Work out the finished part from the listing and answer in its coordinate system (mm). A direction names the side the tool comes from. Coordinates: 2 decimals unless noted, no trailing zeros. Loops run counter-clockwise (first coordinate to the right, second up) from the corner with the lowest first, then second, coordinate; pieces in that order, holes last. Notation, with made-up numbers: M -25,-28 L -17,-28 A27 ccw -17,2 Z; hole C 25.25,57.25 d6. An arc over 180 degrees is marked long. Write each question's results on one line, items separated by ' | '.
```python
from build123d import *

# Parameters (mm, degrees)
CYLINDER883_R               = 1.5
CYLINDER883_DEPTH           = 20
CYLINDER884_R               = 1.5
CYLINDER884_DEPTH           = 20
CYLINDER881_R               = 1.5
CYLINDER881_DEPTH           = 20
CYLINDER885_R               = 1.5
CYLINDER885_DEPTH           = 20
BOX399_W                    = 6
BOX399_H                    = 2
BOX399_DEPTH                = 6
BOX401_W                    = 6
BOX401_H                    = 2
BOX401_DEPTH                = 6
BOX398_W                    = 6
BOX398_H                    = 2
BOX398_DEPTH                = 6
BOX402_W                    = 6
BOX402_H                    = 2
BOX402_DEPTH                = 6
CYLINDER882_R               = 4
CYLINDER882_DEPTH           = 20
CYLINDER882_PLACEMENT_ANGLE = 45
CYLINDER877_R               = 4
CYLINDER877_DEPTH           = 20
CYLINDER877_PLACEMENT_ANGLE = 45
CYLINDER880_R               = 10
CYLINDER880_DEPTH           = 40
CYLINDER878_R               = 10
CYLINDER878_DEPTH           = 40
CYLINDER879_R               = 52
CYLINDER879_DEPTH           = 8
BOX403_W                    = 108
BOX403_H                    = 36
BOX403_DEPTH                = 8
FILLET014_R                 = 12


with BuildPart() as obj1:
    # Cylinder883 → Cylinder883 (new body)
    with BuildSketch(Plane(origin=(24, -40, -5), x_dir=(1, 0, 0), z_dir=(0, -1, 0))):
        Circle(CYLINDER883_R)
    extrude(amount=CYLINDER883_DEPTH)


with BuildPart() as obj2:
    # Cylinder884 → Cylinder884 (new body)
    with BuildSketch(Plane(origin=(51, -40, 7), x_dir=(1, 0, 0), z_dir=(0, -1, 0))):
        Circle(CYLINDER884_R)
    extrude(amount=CYLINDER884_DEPTH)


with BuildPart() as obj3:
    # Cylinder881 → Cylinder881 (new body)
    with BuildSketch(Plane(origin=(-51, -40, 7), x_dir=(1, 0, 0), z_dir=(0, -1, 0))):
        Circle(CYLINDER881_R)
    extrude(amount=CYLINDER881_DEPTH)


with BuildPart() as compound773:
    # Cylinder885 → Cylinder885 (new body)
    with BuildSketch(Plane(origin=(-24, -40, -5), x_dir=(1, 0, 0), z_dir=(0, -1, 0))):
        Circle(CYLINDER885_R)
    extrude(amount=CYLINDER885_DEPTH)

    # Compound773: union obj1, obj2, obj3
    add(obj1.part)
    add(obj2.part)
    add(obj3.part)


with BuildPart() as krychle399:
    # Box399 → Box399 (new body)
    with BuildSketch(Plane(origin=(21, -47, -8), x_dir=(1, 0, 0), z_dir=(0, 0, 1))):
        with Locations((3, 1)):
            Rectangle(BOX399_W, BOX399_H)
    extrude(amount=BOX399_DEPTH)


with BuildPart() as krychle401:
    # Box401 → Box401 (new body)
    with BuildSketch(Plane(origin=(48, -45, 4), x_dir=(1, 0, 0), z_dir=(0, 0, 1))):
        with Locations((3, 1)):
            Rectangle(BOX401_W, BOX401_H)
    extrude(amount=BOX401_DEPTH)


with BuildPart() as krychle398:
    # Box398 → Box398 (new body)
    with BuildSketch(Plane(origin=(-54, -45, 4), x_dir=(1, 0, 0), z_dir=(0, 0, 1))):
        with Locations((3, 1)):
            Rectangle(BOX398_W, BOX398_H)
    extrude(amount=BOX398_DEPTH)


with BuildPart() as compound772:
    # Box402 → Box402 (new body)
    with BuildSketch(Plane(origin=(-27, -47, -8), x_dir=(1, 0, 0), z_dir=(0, 0, 1))):
        with Locations((3, 1)):
            Rectangle(BOX402_W, BOX402_H)
    extrude(amount=BOX402_DEPTH)

    # Compound772: union Krychle399, Krychle401, Krychle398
    add(krychle399.part)
    add(krychle401.part)
    add(krychle398.part)


with BuildPart() as obj4:
    # Cylinder882 → Cylinder882 (new body)
    with BuildSketch(Plane.XY):
        Circle(CYLINDER882_R)
    extrude(amount=CYLINDER882_DEPTH)


with BuildPart() as obj4_1:
    # Cylinder882 placement: moved
    add(obj4.part.moved(Location((39.6, -39.6, -10))).rotate(Axis((39.6, -39.6, -10), (0, 0, 1)), CYLINDER882_PLACEMENT_ANGLE))


with BuildPart() as compound775:
    # Cylinder877 → Cylinder877 (new body)
    with BuildSketch(Plane.XY):
        Circle(CYLINDER877_R)
    extrude(amount=CYLINDER877_DEPTH)


with BuildPart() as compound775_1:
    # Cylinder877 placement: moved
    add(compound775.part.moved(Location((-39.6, -39.6, -10))).rotate(Axis((-39.6, -39.6, -10), (0, 0, -1)), CYLINDER877_PLACEMENT_ANGLE))

    # Compound775: union obj4
    add(obj4_1.part)


with BuildPart() as obj5:
    # Cylinder880 → Cylinder880 (new body)
    with BuildSketch(Plane(origin=(-59, -17, 0), x_dir=(1, 0, 0), z_dir=(0, 0, 1))):
        Circle(CYLINDER880_R)
    extrude(amount=CYLINDER880_DEPTH)


with BuildPart() as compound774:
    # Cylinder878 → Cylinder878 (new body)
    with BuildSketch(Plane(origin=(59, -17, 0), x_dir=(1, 0, 0), z_dir=(0, 0, 1))):
        Circle(CYLINDER878_R)
    extrude(amount=CYLINDER878_DEPTH)

    # Compound774: union obj5
    add(obj5.part)


with BuildPart() as obj6:
    # Cylinder879 → Cylinder879 (new body)
    with BuildSketch(Plane.XY.offset(20)):
        Circle(CYLINDER879_R)
    extrude(amount=CYLINDER879_DEPTH)


with BuildPart() as fillet014:
    # Box403 → Box403 (new body)
    with BuildSketch(Plane(origin=(-54, -53, 20), x_dir=(1, 0, 0), z_dir=(0, 0, 1))):
        with Locations((54, 18)):
            Rectangle(BOX403_W, BOX403_H)
    extrude(amount=BOX403_DEPTH)

    # Cut400: cut obj6
    add(obj6.part, mode=Mode.SUBTRACT)


with BuildPart() as fillet014_1:
    # Cut400 placement: moved
    add(fillet014.part.moved(Location((0, 0, -20))))

    # Cut403: cut Compound774
    add(compound774.part, mode=Mode.SUBTRACT)


with BuildPart() as fillet014_2:
    # Cut403 placement: moved
    add(fillet014_1.part.moved(Location((0, 0, -8))))

    # Cut401: cut Compound775
    add(compound775_1.part, mode=Mode.SUBTRACT)

    # Cut402: cut Compound772
    add(compound772.part, mode=Mode.SUBTRACT)

    # Cut399: cut Compound773
    add(compound773.part, mode=Mode.SUBTRACT)

    # Fillet014
    fillet014_edges = [fillet014_2.edges().sort_by_distance(p)[0] for p in [
        (-54, -25.660254, -4),
        (54, -25.660254, -4),
    ]]
    fillet(fillet014_edges, radius=FILLET014_R)


solid = fillet014_2.part
```
1) Straight lines are drawn through the part: probe 1 along X at (y, z) = (-39.6, -5.25); probe 2 along X at (y, z) = (-48, -5.75); probe 3 along X at (y, z) = (-20.5, -3.5). For each, find the intervals that lie inside material, in ascending order. Write a range as [from, to].
Check result:
probe 1: [-54, -43.6], [-35.6, -33.7], [33.7, 35.6], [43.6, 54] | probe 2: [-54, -25.3], [-22.7, -20], [20, 22.7], [25.3, 54] | probe 3: [-49.63, -47.79], [47.79, 49.63]
2) For a pull along X with two mould halves and no side action, classify faces 1 (the face through (-38.071, -43.296, -4.056)), 2 (the face through (54, -42, -4)), 3 (the face through (-54, -42, -4)) as released by +X, released by -X, zero draft, split by the parting line, or undercut.
Check result:
face 1: undercut | face 2: released by +X | face 3: released by -X
3) Given pin 1 Ø1.4 at (x, z) = (25, -4.5) entering from +Y; pin 2 Ø0.6 at (x, y) = (25.5, -46) entering from -Z, each flat-ended and moving along its own axis, determine where each tip first touches the part or whether it passes through.
Check result:
pin 1: y = -47 | pin 2: z = -2
4) Find section B-B, the plane y = -27.5. Give the vertices of the cut face in (x, z).
Check result:
outline: M -53.49,-8 L -44.13,-8 L -44.13,0 L -53.49,0 Z; M 44.13,-8 L 53.49,-8 L 53.49,0 L 44.13,0 Z
5) Find section A-A, the plane x = 24. Give the vertices of the cut face in (y, z).
Check result:
outline: M -53,-8 L -47,-8 L -47,-6.5 L -53,-6.5 Z; M -53,-3.5 L -47,-3.5 L -47,-2 L -46.13,-2 L -46.13,0 L -53,0 Z
6) Which of the six approach directions +Z, -Z, +X, -X, +Y, -Y give full straight-line access (tool end or side, diameter ignored) to faces 4 (the face through (-25, -46, -2)), 5 (the face through (-4, -52, -8))?
Check result:
face 4: -Z | face 5: -Z, +X, -X, +Y, -Y
7) Find section D-D, the plane y = -39.6. Give the vertices of the cut face in (x, z), and give its area (3 significant figures).
Check result:
outline: M -54,-8 L -43.6,-8 L -43.6,0 L -54,0 Z; M -35.6,-8 L -33.7,-8 L -33.7,0 L -35.6,0 Z; M 33.7,-8 L 35.6,-8 L 35.6,0 L 33.7,0 Z; M 43.6,-8 L 54,-8 L 54,0 L 43.6,0 Z | area: 197 mm^2
8) Find section C-C, the plane z = -5. Give the vertices of the cut face in (x, y).
Check result:
outline: M -54,-53 L -25.5,-53 L -25.5,-47 L -27,-47 L -27,-45 L -26.06,-45 A52 cw -49.01,-17.39 A10 cw -51.27,-23.35 A12 ccw -54,-30.96 Z; M -22.5,-53 L 22.5,-53 L 22.5,-47 L 22.25,-47 A52 cw -22.25,-47 L -22.5,-47 Z; M 25.5,-53 L 54,-53 L 54,-30.96 A12 ccw 51.27,-23.35 A10 cw 49.01,-17.39 A52 cw 26.06,-45 L 27,-45 L 27,-47 L 25.5,-47 Z; hole C -39.6,-39.6 d8; hole C 39.6,-39.6 d8
